from build123d import *

# Parameters (mm, degrees)
F0_W     = 35
F0_H     = 100
F1_DEPTH = 3
F2_W     = 35
F2_H     = 35
F3_DEPTH = 6
F4_R     = 2.625
F5_DEPTH = 4
F6_W     = 8
F6_H     = 8
F6_W_2   = 5
F6_H_2   = 5
F7_DEPTH = 6


with BuildPart() as f1:
    # F0 (on Top) → F1 (new body)
    with BuildSketch(Plane.XY):
        Rectangle(F0_W, F0_H)
    extrude(amount=F1_DEPTH)

    # F2 (on face) → F3 (join)
    with BuildSketch(Plane.XY.offset(3)):
        Rectangle(F2_W, F2_H)
    extrude(amount=F3_DEPTH)

    # F4 (on face) → F5 (cut)
    with BuildSketch(Plane.XY.offset(9)):
        Circle(F4_R)
    extrude(amount=-F5_DEPTH, mode=Mode.SUBTRACT)

    # F6 (on face) → F7 (join)
    with BuildSketch(Plane.XY.offset(3)):
        with Locations((0, 35.393093)):
            Rectangle(F6_W, F6_H)
        with Locations((0, 35.393093)):
            Rectangle(F6_W_2, F6_H_2, mode=Mode.SUBTRACT)
    extrude(amount=F7_DEPTH)


solid = f1.part
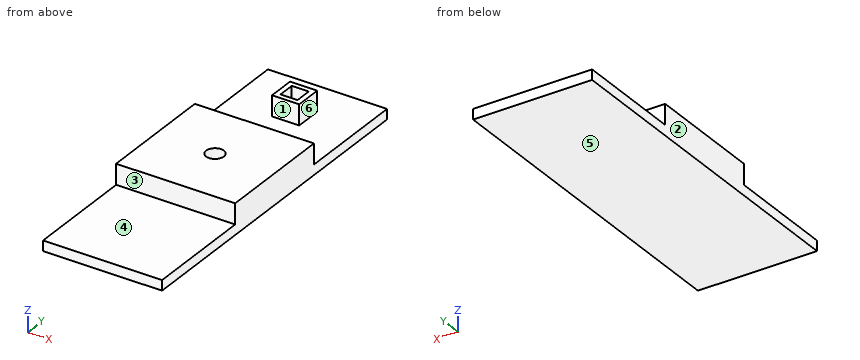
Geometry: final body of the model. Coordinates: model frame, mm. Face numbers are marked on the shaded views. A direction names the side the tool comes from. Give positions to 0.01 mm unless a question says otherwise; leave off trailing zeros. Write each loop counter-clockwise with the first axis right and the second up, starting at its lowest first coordinate (ties: lowest second). Pieces come first, ordered by that corner, then holes. Notation, with made-up numbers: M 18,69.5 L 53,69.5 A13 ccw 53,73.5 Z; hole C -38.75,43 d10. An arc over 180 degrees is marked long. Answer in a Markdown table with one row per item. Add a question column.
(1) First-contact query: pin 1 (1.8 mm diameter, centred on x = -8, z = 5, fed in from +Y); pin 2 (4 mm diameter, centred on x = 0, y = 0, fed in from +Z); pin 3 (5 mm diameter, centred on x = 1.5, z = 6, fed in from +Y); pin 4 (1 mm diameter, centred on y = 29, z = 8, fed in from -X). Flat tips, straight axial feed; report the tip coordinate or a pass-through.
(2) Section D-D on y = 0. Return loops of the section in (x, z) (3 decimals), and give its area (3 significant figures).
(3) Section B-B on x = 0. Return loops of the section in (y, z) (3 decimals), and give its area (3 significant figures).
(4) Reachability of the marked faces 4, 5 and 6 from +Z, -Z, +X, -X, +Y, -Y: full face, straight path, thin tool, end or side. Return the list, or none.
(5) Mould query, pull axis Y, two halves, no side actions, for the marked faces 1, 2 and 3. Classes: +Y half, -Y half, draft (parallel to the pull), parting line (faces both ways), or undercut.
(6) Section C-C on y = 34.5. Return loops of the section in (x, z), and give its area (3 significant figures).
(7) Ray query, line 1 (Y direction, x = 0, z = 8.05) (3 decimals); line 2 (X direction, y = 35.5, z = 7.5); line 3 (Z direction, x = 6.5, y = -25.5). Return the intervals inside material, ascending.
(8) Section A-A on z = 7. Return loops of the section in (x, y) (3 decimals), and give its area (3 significant figures).
Result set:
| question | item | result |
|---|---|---|
| 1 | pin 1 | stops at y = 17.5 |
| 1 | pin 2 | stops at z = 5 |
| 1 | pin 3 | stops at y = 39.39 |
| 1 | pin 4 | passes through |
| 2 | outline | M -17.5,0 L 17.5,0 L 17.5,9 L 2.625,9 L 2.625,5 L -2.625,5 L -2.625,9 L -17.5,9 Z |
| 2 | area | 294 mm^2 |
| 3 | outline | M -50,0 L 50,0 L 50,3 L 39.393,3 L 39.393,9 L 37.893,9 L 37.893,3 L 32.893,3 L 32.893,9 L 31.393,9 L 31.393,3 L 17.5,3 L 17.5,9 L 2.625,9 L 2.625,5 L -2.625,5 L -2.625,9 L -17.5,9 L -17.5,3 L -50,3 Z |
| 3 | area | 507 mm^2 |
| 4 | face 4 | +Z, +X, -X, -Y |
| 4 | face 5 | -Z, +X, -X, +Y, -Y |
| 4 | face 6 | +Z, +X, +Y |
| 5 | face 1 | undercut |
| 5 | face 2 | draft |
| 5 | face 3 | -Y half |
| 6 | outline | M -17.5,0 L 17.5,0 L 17.5,3 L 4,3 L 4,9 L 2.5,9 L 2.5,3 L -2.5,3 L -2.5,9 L -4,9 L -4,3 L -17.5,3 Z |
| 6 | area | 123 mm^2 |
| 7 | line 1 | y = -17.5 to -2.625, 2.625 to 17.5, 31.393 to 32.893, 37.893 to 39.393 |
| 7 | line 2 | x = -4 to -2.5, 2.5 to 4 |
| 7 | line 3 | z = 0 to 3 |
| 8 | outline | M -17.5,-17.5 L 17.5,-17.5 L 17.5,17.5 L -17.5,17.5 Z; M -4,31.393 L 4,31.393 L 4,39.393 L -4,39.393 Z; hole C 0,0 d5.25; hole M -2.5,32.893 L 2.5,32.893 L 2.5,37.893 L -2.5,37.893 Z |
| 8 | area | 1,240 mm^2 |
